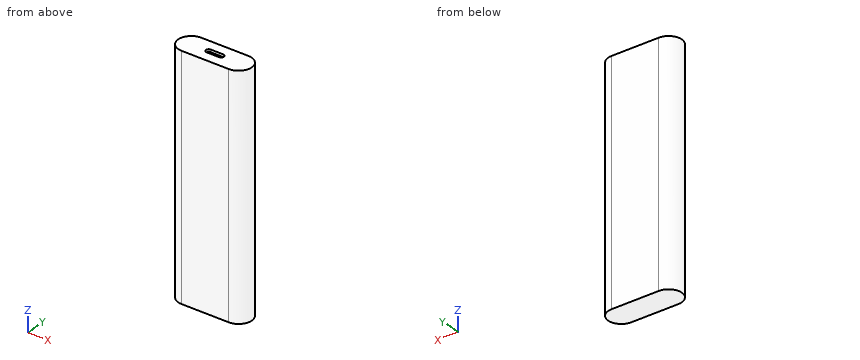
from build123d import *

# Parameters (mm, degrees)
BOSS_EXTRUDE1_DEPTH = 107.7
CUT_EXTRUDE1_DEPTH  = 6.5
SKETCH3_W           = 6.69
SKETCH3_H           = 0.8
BOSS_EXTRUDE2_DEPTH = 6


with BuildPart() as part:
    # Sketch1 → Boss-Extrude1 (new body)
    with BuildSketch(Plane.XY):
        with BuildLine():
            Line((-10.95, 6), (10.95, 6))
            ThreePointArc((10.95, 6), (16.95, 0), (10.95, -6))
            Line((10.95, -6), (-10.95, -6))
            ThreePointArc((-10.95, -6), (-16.95, 0), (-10.95, 6))
        make_face()
    extrude(amount=-BOSS_EXTRUDE1_DEPTH)

    # Sketch2 → Cut-Extrude1 (cut)
    with BuildSketch(Plane.XY):
        with BuildLine():
            Line((-2.89, 1.28), (2.89, 1.28))
            ThreePointArc((2.89, 1.28), (4.17, 0), (2.89, -1.28))
            Line((2.89, -1.28), (-2.89, -1.28))
            ThreePointArc((-2.89, -1.28), (-4.17, 0), (-2.89, 1.28))
        make_face()
    extrude(amount=-CUT_EXTRUDE1_DEPTH, mode=Mode.SUBTRACT)

    # Sketch3 → Boss-Extrude2 (add)
    with BuildSketch(Plane.XY.offset(-6.5)):
        Rectangle(SKETCH3_W, SKETCH3_H)
    extrude(amount=BOSS_EXTRUDE2_DEPTH)


solid = part.part
Verification items for the finished model (mm, model axes). Give positions to 0.01 mm unless a question says otherwise; leave off trailing zeros. Write each loop counter-clockwise with the first axis right and the second up, starting at its lowest first coordinate (ties: lowest second). Pieces come first, ordered by that corner, then holes. Notation, with made-up numbers: M 83.25,13.25 L 103.25,13.25 A30 ccw 103.25,46.25 Z; hole C 10.5,26.25 d3. An arc over 180 degrees is marked long. Put each result on its own line as item: value. Start each with the question number.
1. Section check B-B (y = 3). Record the cut outline in (x, z), and give its area (3 significant figures).
2. Scan lines: line 1 along X through (y, z) = (0.25, -53); line 2 along Y through (x, z) = (-14, -88); line 3 along X through (y, z) = (4.25, -80.5). Record each from-to range of solid material in increasing order. Write a range as [from, to].
3. Go/stop test with flat-tipped pins: pin 1 Ø1 at (y, z) = (3.5, -56) entering from -X; pin 2 Ø2 at (x, y) = (0.5, 0) entering from +Z. Record where each tip stops, or that it passes through.
4. Section check A-A (z = -94). Record the cut outline in (x, y), and give its area (3 significant figures).
Answer list:
1. outline: M -16.15,-107.7 L 16.15,-107.7 L 16.15,0 L -16.15,0 Z
1. area: 3,480 mm2
2. line 1: [-16.94, 16.94]
2. line 2: [-5.17, 5.17]
2. line 3: [-15.19, 15.19]
3. pin 1: x = -16.15
3. pin 2: z = -0.5
4. outline: M -10.95,-6 L 10.95,-6 A6 ccw 10.95,6 L -10.95,6 A6 ccw Z
4. area: 376 mm2
